```python
from build123d import *

# Parameters (mm, degrees)
F0_W     = 60
F0_H     = 20
F1_DEPTH = 20
F2_W     = 20
F2_H     = 60
F3_DEPTH = 20
F4_W     = 10
F4_H     = 40
F5_DEPTH = 10
F7_DEPTH = 10
F8_SIZE  = 10
F9_SIZE  = 5
F10_SIZE = 5


with BuildPart() as f1:
    # F0 (on Top) → F1 (new body)
    with BuildSketch(Plane.XY):
        with Locations((30, 10)):
            Rectangle(F0_W, F0_H)
    extrude(amount=F1_DEPTH)

    # F2 (on Front) → F3 (join)
    with BuildSketch(Plane.XZ):
        with Locations((10, 30)):
            Rectangle(F2_W, F2_H)
    extrude(amount=-F3_DEPTH)

    # F4 (on face) → F5 (cut)
    with BuildSketch(Plane.YZ.offset(20)):
        with Locations((10.1094414666, 40)):
            Rectangle(F4_W, F4_H)
    extrude(amount=-F5_DEPTH, mode=Mode.SUBTRACT)

    # F6 (on face) → F7 (cut)
    with BuildSketch(Plane.XY.offset(20)):
        Polygon((20, 15.1094414666), (10, 15.1094414666), (10, 5.1094414666), (20, 5.1094414666), (60, 5.1094414666), (60, 15.1094414666), align=None)
    extrude(amount=-F7_DEPTH, mode=Mode.SUBTRACT)

    # F8
    f8_edges = [f1.edges().sort_by_distance(p)[0] for p in [
        (0, 10, 0),
    ]]
    chamfer(f8_edges, length=F8_SIZE)

    # F9
    f9_edges = [f1.edges().sort_by_distance(p)[0] for p in [
        (35, 0, 0),
        (5, 0, 5),
    ]]
    chamfer(f9_edges, length=F9_SIZE)

    # F10
    f10_edges = [f1.edges().sort_by_distance(p)[0] for p in [
        (0, 0, 38.535534),
    ]]
    chamfer(f10_edges, length=F10_SIZE)


solid = f1.part
```
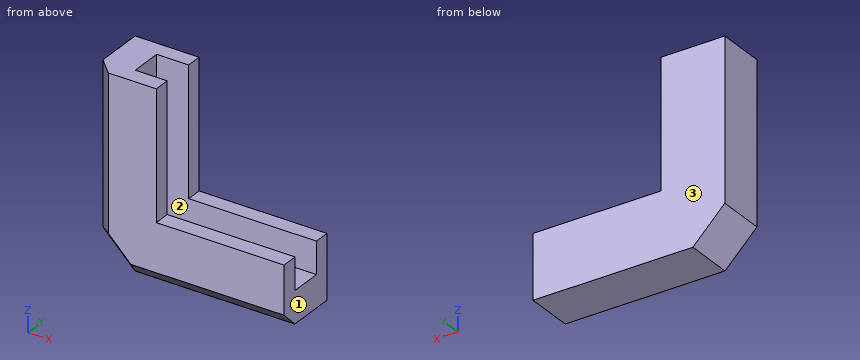
Here's how the part is built. I have some questions about the finished solid (model axes, mm). Face numbers are marked on the shaded views. Coordinates: 2 decimals unless noted, no trailing zeros. Loops run counter-clockwise (first coordinate to the right, second up) from the corner with the lowest first, then second, coordinate; pieces in that order, holes last. Notation, with made-up numbers: (-39, 44) - (-2, 44) arc R27 cw to (-2, 71) - close; hole circle Ø10 at (76.5, -25.75). An arc over 180 degrees is marked (long way). Return JSON: item names as keys, results as strings. Group by question number.
Item 1: We'd pull the mould along Y, two halves only. Please class the marked faces 1, 2 and 3: +Y half, -Y half, draft (parallel to the pull), parting line (faces both ways), or undercut.
Item 2: If we section it at B-B on x = 15: Write out the boundary of the cut face in (y, z).
Item 3: If we section it at A-A on z = 13.5: Write out the boundary of the cut face in (x, y), and give its area (4 significant figures).
Item 4: If we section it at C-C on y = 12.5: Write out the boundary of the cut face in (x, z).
Item 5: Will these pins go through, and if not, where does the flat tip stop? P1, Ø2.5, axis at x = 31, y = 17.5, coming from the +Z side; P2, Ø1, axis at y = 9, z = 32.5, coming from the +X side; P3, Ø5, axis at x = 51.5, y = 12, coming from the +Z side.
Item 6: If we section it at D-D on y = 18: Write out the boundary of the cut face in (x, z).
Item 7: I need wall thicknesses on line 1 (Z direction, x = 40.5, y = 5); line 2 (Y direction, x = 37, z = 18.5). Which ranges of each line are inside material? Lowest first, please. Write a range as from..to.
Calculated:
{
 "1": {"face 1": "draft", "face 2": "undercut", "face 3": "+Y half"},
 "2": {"outline": "(0, 5) - (5, 0) - (20, 0) - (20, 60) - (15.11, 60) - (15.11, 10) - (5.11, 10) - (5.11, 60) - (0, 60) - close"},
 "3": {"outline": "(0, 5) - (5, 0) - (60, 0) - (60, 5.11) - (10, 5.11) - (10, 15.11) - (60, 15.11) - (60, 20) - (0, 20) - close", "area": "687.5 mm^2"},
 "4": {"outline": "(0, 10) - (10, 0) - (60, 0) - (60, 10) - (10, 10) - (10, 60) - (0, 60) - close"},
 "5": {"P1": "stops at z = 20", "P2": "stops at x = 10", "P3": "stops at z = 10"},
 "6": {"outline": "(0, 10) - (10, 0) - (60, 0) - (60, 20) - (20, 20) - (20, 60) - (0, 60) - close"},
 "7": {"line 1": "z = 0..20", "line 2": "y = 0..5.11, 15.11..20"}
}
